Build history of the part. All positions in model axes, mm. Face numbers are marked on the shaded views. Round coordinates to 2 decimals unless told otherwise and drop trailing zeros. Loops run counter-clockwise (first coordinate to the right, second up) from the corner with the lowest first, then second, coordinate; pieces in that order, holes last.
Autodesk Inventor part; units mm, degrees
ref_plane "YZ Plane" through (0, 0, 0) normal (1, 0, 0) x (0, 1, 0)
ref_plane "XZ Plane" through (0, 0, 0) normal (0, 1, 0) x (-1, 0, 0)
ref_plane "XY Plane" through (0, 0, 0) normal (0, 0, 1) x (1, 0, 0)
sketch "Sketch2" plane through (0, 0, 0) normal (0, 0, 1) x (1, 0, 0)
  line L0 (-75, -25) -> (75, -25)
  line L1 (75, -25) -> (75, 25)
  line L2 (75, 25) -> (-75, 25)
  line L3 (-75, 25) -> (-75, -25)
  line L4 (-75, -25) -> (75, 25) construction
  line L5 (75, -25) -> (-75, 25) construction
  point P0 (0, 0)
  dimension "d1" = 150
  dimension "d2" = 50
extrude "Extrusion1" add sketch "Sketch2" along normal mid plane 10
sketch "Sketch3" plane through (0, 0, 5) normal (0, 0, 1) x (1, 0, 0)
  line L0 (-75, 25) -> (-75, -25)
  line L1 (75, 25) -> (-75, 25)
  point P0 (0, 0)
  point P1 (-65, 0)
  dimension "d40" = 10
  dimension "d43" = 25
hole "Hole1" at (-65, 0, 5) direction (0, 0, -1) diameter 5.5 depth 14.2 tip angle 118
sketch "Sketch4" plane through (0, 0, 5) normal (0, 0, 1) x (1, 0, 0)
  line L0 (-75, 25) -> (-75, -25)
  line L1 (75, 25) -> (-75, 25)
  point P0 (0, 0)
  point P1 (-45, 5)
  dimension "d41" = 30
  dimension "d42" = 20
hole "Hole2" at (-45, 5, 5) direction (0, 0, -1) diameter 6.6 depth 14.2 tip angle 118
sketch "Sketch5" plane through (0, 0, 5) normal (0, 0, 1) x (1, 0, 0)
  line L0 (-75, 25) -> (-75, -25)
  line L1 (75, 25) -> (-75, 25)
  point P0 (0, 0)
  point P1 (-25, 5)
  dimension "d44" = 50
  dimension "d45" = 20
hole "Hole3" at (-25, 5, 5) direction (0, 0, -1) diameter 9 depth 14.2 tip angle 118
sketch "Sketch6" plane through (0, 0, 5) normal (0, 0, 1) x (1, 0, 0)
  line L0 (-75, 25) -> (-75, -25)
  line L1 (75, 25) -> (-75, 25)
  point P0 (0, 0)
  point P1 (5, 5)
  dimension "d46" = 80
  dimension "d47" = 20
hole "Hole4" at (5, 5, 5) direction (0, 0, -1) diameter 6 depth 14.2 tip angle 118
sketch "Sketch7" plane through (0, 0, 5) normal (0, 0, 1) x (1, 0, 0)
  line L0 (-75, 25) -> (-75, -25)
  line L1 (75, 25) -> (-75, 25)
  point P0 (0, 0)
  point P1 (25, 5)
  dimension "d48" = 100
  dimension "d49" = 20
hole "Hole5" at (25, 5, 5) direction (0, 0, -1) diameter 10 depth 14.2 tip angle 118
sketch "Sketch8" plane through (0, 0, 5) normal (0, 0, 1) x (1, 0, 0)
  point P0 (0, 0)
  point P1 (51.0965, 5.234)
hole "Hole6" at (51.0965, 5.234, 5) direction (0, 0, -1) diameter 21 depth 14.2 tip angle 118
properties part number "홀간 거리 확인 파트-1" material "SS400"
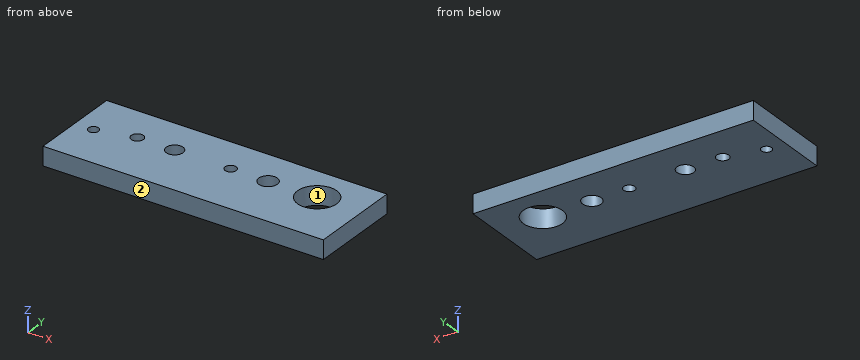
(1) Probe line 1 (X direction, y = 5, z = -1.25); line 2 (X direction, y = 1.5, z = 1.5); line 3 (Y direction, x = 5, z = -1.5). List the from-to ranges inside material, lowest first.
Responses:
line 1: x = -75 to -48.3, -41.7 to -29.5, -20.5 to 2, 8 to 20, 30 to 40.6, 61.59 to 75
line 2: x = -75 to -67.3, -62.7 to -27.83, -22.17 to 21.43, 28.57 to 41.28, 60.91 to 75
line 3: y = -25 to 2, 8 to 25
(2) Slice it at B-B on z = -2.5. List the corners of the cut face in (x, y), plus the area to 3 significant figures.
Responses:
outline: (-75, -25) - (75, -25) - (75, 25) - (-75, 25) - close; hole circle Ø5.5 at (-65, 0); hole circle Ø6.6 at (-45, 5); hole circle Ø9 at (-25, 5); hole circle Ø6 at (5, 5); hole circle Ø10 at (25, 5); hole circle Ø21 at (51.1, 5.23)
area: 6,930 mm2
(3) Pull direction X, two halves, no side cores. Call the marked faces 1 and 2: +X half, -X half, draft (parallel to the pull), parting line (faces both ways), or undercut.
Responses:
face 1: undercut
face 2: draft
(4) Slice it at C-C on x = 25. List the corners of the cut face in (y, z).
Responses:
outline: (-25, -5) - (0, -5) - (0, 5) - (-25, 5) - close; (10, -5) - (25, -5) - (25, 5) - (10, 5) - close
(5) Pin check, flat tip, straight feed: P1, Ø5.5, axis at x = -25, y = 5, coming from the +Z side. Stop position of the tip, or through.
Responses:
P1: passes through
(6) Slice it at A-A on x = -45. List the corners of the cut face in (y, z).
Responses:
outline: (-25, -5) - (1.7, -5) - (1.7, 5) - (-25, 5) - close; (8.3, -5) - (25, -5) - (25, 5) - (8.3, 5) - close
(7) Slice it at D-D on y = 5. List the corners of the cut face in (x, z).
Responses:
outline: (-75, -5) - (-48.3, -5) - (-48.3, 5) - (-75, 5) - close; (-41.7, -5) - (-29.5, -5) - (-29.5, 5) - (-41.7, 5) - close; (-20.5, -5) - (2, -5) - (2, 5) - (-20.5, 5) - close; (8, -5) - (20, -5) - (20, 5) - (8, 5) - close; (30, -5) - (40.6, -5) - (40.6, 5) - (30, 5) - close; (61.59, -5) - (75, -5) - (75, 5) - (61.59, 5) - close
